Source: CAD feature listing. Evaluate the final solid. Frame: model axes, mm. A direction names the side the tool comes from. Round coordinates to 2 decimals unless told otherwise and drop trailing zeros. Order: outer loops, then holes, each group sorted by start corner. A loop starts at its lowest first (then second) coordinate and runs counter-clockwise, first axis right, second up.
```python
from build123d import *

# Parameters (mm, degrees)
F0_W      = 5
F0_H      = 4
F1_DEPTH  = 6
F2_W      = 4
F2_H      = 2
F3_DEPTH  = 6.001
F4_W      = 0.75
F4_H      = 0.5
F5_DEPTH  = 6.001
F6_W      = 3
F6_H      = 0.5
F7_DEPTH  = 5.001
F8_R      = 1.5
F9_DEPTH  = 1.001
F10_R     = 0.5
F11_R     = 0.25
F12_DEPTH = 2.001


# Not quite as in the source:
# - a pattern or mirror of a feature is missing from the dataset's text; its kind, count and spacing are read off the source's solid


with BuildPart() as f1:
    # F0 (on Front) → F1 (new body)
    with BuildSketch(Plane.XZ):
        Rectangle(F0_W, F0_H)
    extrude(amount=F1_DEPTH)

    # F2 (on face) → F3 (cut, through all)
    with BuildSketch(Plane.XZ.offset(6)):
        with Locations((-0.5, 1)):
            Rectangle(F2_W, F2_H)
    extrude(amount=-F3_DEPTH, mode=Mode.SUBTRACT)

    # F4 (on face) → F5 (cut, through all)
    with BuildSketch(Plane.XZ.offset(6)):
        with Locations((0, -0.25)):
            Rectangle(F4_W, F4_H)
        Polygon((1, -0.5), (0.375, -0.5), (-0.375, -0.5), (-1, -0.5), (-1, -1), (1, -1), align=None)
    extrude(amount=-F5_DEPTH, mode=Mode.SUBTRACT)

    # F6 (on face) → F7 (cut, through all)
    with BuildSketch(Plane(origin=(-2.5, 0, 0), x_dir=(0, -1, 0), z_dir=(-1, 0, 0))):
        with Locations((3, -1.75)):
            Rectangle(F6_W, F6_H)
    extrude(amount=-F7_DEPTH, mode=Mode.SUBTRACT)

    # F8 (on face) → F9 (cut, through all)
    with BuildSketch(Plane(origin=(1.5, 0, 0), x_dir=(0, -1, 0), z_dir=(-1, 0, 0))):
        with Locations((3, 2)):
            Circle(F8_R)
    extrude(amount=-F9_DEPTH, mode=Mode.SUBTRACT)

    # F10
    f10_edges = [f1.edges().sort_by_distance(p)[0] for p in [
        (2, -6, 2),
        (2, 0, 2),
    ]]
    fillet(f10_edges, radius=F10_R)

    # F11 (on face) → F12 (cut, through all)
    with BuildSketch(Plane.XY):
        with Locations((-1.75, -0.75)):
            Circle(F11_R)
    f12 = extrude(amount=-F12_DEPTH, mode=Mode.SUBTRACT)

    # F12_copies: F12 across plane
    add(f12.mirror(Plane(origin=(0, -3, 0), x_dir=(0, 0, -1), z_dir=(0, -1, 0))), mode=Mode.SUBTRACT)


solid = f1.part
```
1. Line query: line 1 along Y through (x, z) = (-1.75, -1.4); line 2 along X through (y, z) = (-5.25, -0.7); line 3 along Y through (x, z) = (0.3, -1.6). Output: solid intervals per line, ascending.
2. Access query for faces 4 (the face through (0, -3, -1.5)), 5 (the face through (-1, -3, 0)), 6 (the face through (0, -3, -1)). Directions: +Z, -Z, +X, -X, +Y, -Y. A direction counts if a zero-diameter tool reaches every point of the face in a straight line with its end or side. Return the directions, or none.
3. Section A-A on z = -1.7. Return loops of the section in (x, y).
4. Pull-direction query (Y, two-part tool) for faces 1 (the face through (2, -3, 0.5)), 2 (the face through (0.5, -6, -1.4)), 3 (the face through (2, -5, 2)); classes: released by +Y, released by -Y, zero draft, split by the parting line, or undercut.
5. Section D-D on z = 1.65. Return loops of the section in (x, y), plus the area to 3 significant figures.
6. Section C-C on x = -0.8. Return loops of the section in (y, z), plus the area to 3 significant figures.
7. First-contact query: pin 1 (1.7 mm diameter, centred on x = -2, y = -3.5, fed in from +Z); pin 2 (0.5 mm diameter, centred on x = -0.5, y = -3, fed in from -Z). Flat tips, straight axial feed; report the tip coordinate or a pass-through.
8. Section B-B on y = -5.25. Return loops of the section in (x, z) (3 decimals).
Result:
1. line 1: y = -6 to -5.5, -5 to -1, -0.5 to 0
1. line 2: x = -2.5 to -2, -1.5 to -1, 1 to 2.5
1. line 3: y = -6 to -4.5, -1.5 to 0
2. face 4: -Z, +X, -X
2. face 5: +Z, -X, +Y, -Y
2. face 6: +Y, -Y
3. outline: (-2.5, -6) - (2.5, -6) - (2.5, -4.5) - (-2.5, -4.5) - close; (-2.5, -1.5) - (2.5, -1.5) - (2.5, 0) - (-2.5, 0) - close; hole circle Ø0.5 at (-1.75, -5.25); hole circle Ø0.5 at (-1.75, -0.75)
4. face 1: undercut
4. face 2: released by -Y
4. face 3: zero draft
5. outline: (1.5, -5.98) - (2.5, -5.98) - (2.5, -4.46) - (1.5, -4.46) - close; (1.5, -1.54) - (2.5, -1.54) - (2.5, -0.02) - (1.5, -0.02) - close
5. area: 3.04 mm2
6. outline: (-6, -2) - (-4.5, -2) - (-4.5, -1.5) - (-1.5, -1.5) - (-1.5, -2) - (0, -2) - (0, -1) - (-6, -1) - close; (-6, -0.5) - (0, -0.5) - (0, 0) - (-6, 0) - close
6. area: 7.50 mm2
7. pin 1: stops at z = 0
7. pin 2: stops at z = -1.5
8. outline: (-2.5, -2) - (-2, -2) - (-2, 0) - (-2.5, 0) - close; (-1.5, -2) - (2.5, -2) - (2.5, 2) - (1.5, 2) - (1.5, 0) - (0.375, 0) - (0.375, -0.5) - (1, -0.5) - (1, -1) - (-1, -1) - (-1, -0.5) - (-0.375, -0.5) - (-0.375, 0) - (-1.5, 0) - close
